```python
from build123d import *

# Parameters (mm, degrees)
SKETCH1_R           = 2.5
BOSS_EXTRUDE5_DEPTH = 2.5
SKETCH7_R           = 20
BOSS_EXTRUDE6_DEPTH = 1.5
CUT_EXTRUDE5_DEPTH  = 3
SKETCH9_R           = 30
SKETCH9_R_2         = 20
BOSS_EXTRUDE8_DEPTH = 2
SKETCH10_R          = 1.5
CUT_EXTRUDE6_DEPTH  = 2
CUT_EXTRUDE7_DEPTH  = 2
FILLET1_R           = 1
FILLET2_R           = 1


# Some blends are built 0.0001 mm under size
with BuildPart() as part:
    # Sketch1 → Boss-Extrude5 (new, symmetric)
    with BuildSketch(Plane.XY):
        Circle(SKETCH1_R)
    extrude(amount=BOSS_EXTRUDE5_DEPTH, both=True)

    # Sketch7 → Boss-Extrude6 (add, symmetric)
    with BuildSketch(Plane.XY):
        Circle(SKETCH7_R)
    extrude(amount=BOSS_EXTRUDE6_DEPTH, both=True)

    # Sketch8 → Cut-Extrude5 (cut)
    with BuildSketch(Plane.XY.offset(1.5)):
        with BuildLine():
            Line((0, 2.5), (0, 17.5))
            ThreePointArc((0, 17.5), (3.385621722, 10), (0, 2.5))
        make_face()
        with BuildLine():
            Line((1.767766953, 1.767766953), (12.374368671, 12.374368671))
            ThreePointArc((12.374368671, 12.374368671), (9.46506389, 4.677071733), (1.767766953, 1.767766953))
        make_face()
        with BuildLine():
            Line((2.5, 0), (17.5, 0))
            ThreePointArc((17.5, 0), (10, -3.385621722), (2.5, 0))
        make_face()
        with BuildLine():
            Line((1.767766953, -1.767766953), (12.374368671, -12.374368671))
            ThreePointArc((12.374368671, -12.374368671), (4.677071733, -9.46506389), (1.767766953, -1.767766953))
        make_face()
        with BuildLine():
            Line((0, -2.5), (0, -17.5))
            ThreePointArc((0, -17.5), (-3.385621722, -10), (0, -2.5))
        make_face()
        with BuildLine():
            Line((-1.767766953, -1.767766953), (-12.374368671, -12.374368671))
            ThreePointArc((-12.374368671, -12.374368671), (-9.46506389, -4.677071733), (-1.767766953, -1.767766953))
        make_face()
        with BuildLine():
            Line((-2.5, 0), (-17.5, 0))
            ThreePointArc((-17.5, 0), (-10, 3.385621722), (-2.5, 0))
        make_face()
        with BuildLine():
            Line((-1.767766953, 1.767766953), (-12.374368671, 12.374368671))
            ThreePointArc((-12.374368671, 12.374368671), (-4.677071733, 9.46506389), (-1.767766953, 1.767766953))
        make_face()
    extrude(amount=-CUT_EXTRUDE5_DEPTH, mode=Mode.SUBTRACT)

    # Sketch9 → Boss-Extrude8 (add, symmetric)
    with BuildSketch(Plane.XY):
        Circle(SKETCH9_R)
        Circle(SKETCH9_R_2, mode=Mode.SUBTRACT)
    extrude(amount=BOSS_EXTRUDE8_DEPTH, both=True)

    # Sketch10 → Cut-Extrude6 (cut)
    with BuildSketch(Plane.XY.offset(2.5)):
        Circle(SKETCH10_R)
    extrude(amount=-CUT_EXTRUDE6_DEPTH, mode=Mode.SUBTRACT)

    # Sketch11 → Cut-Extrude7 (cut)
    with BuildSketch(Plane.XY.offset(0.5)):
        with BuildLine():
            Line((-1.5, 0), (1.5, 0))
            ThreePointArc((1.5, 0), (0, -1.5), (-1.5, 0))
        make_face()
    extrude(amount=-CUT_EXTRUDE7_DEPTH, mode=Mode.SUBTRACT)

    # Fillet1
    fillet1_edges = [part.edges().sort_by_distance(p)[0] for p in [
        (-2.5, 0, -2.5),
    ]]
    fillet(fillet1_edges, radius=FILLET1_R - 0.0001)  # a hair under: the kernel refuses the full size

    # Fillet2
    # the kernel refuses this fillet: 1 mm, written as the material it takes off along each edge
    with BuildSketch(Plane(origin=(0, 0, 2), x_dir=(1, 0, 0), z_dir=(0, -1, 0))) as fillet2_piece_1:
        with BuildLine():
            CenterArc((30 - FILLET2_R, -FILLET2_R), FILLET2_R, 0, 90)
            Line((30 - FILLET2_R, 0), (30 - FILLET2_R, FILLET2_R * 0.02))
            Line((30 - FILLET2_R, FILLET2_R * 0.02), (30 + FILLET2_R * 0.02, FILLET2_R * 0.02))
            Line((30 + FILLET2_R * 0.02, FILLET2_R * 0.02), (30 + FILLET2_R * 0.02, -FILLET2_R))
            Line((30 + FILLET2_R * 0.02, -FILLET2_R), (30, -FILLET2_R))
        make_face()
    revolve(axis=Axis((0, 0, 2), (0, 0, 1)), mode=Mode.SUBTRACT)
    with BuildSketch(Plane(origin=(0, 0, -2), x_dir=(1, 0, 0), z_dir=(0, -1, 0))) as fillet2_piece_2:
        with BuildLine():
            CenterArc((20.866025404, 1), FILLET2_R, 210, 60)
            Line((20.866025404, 0), (20.866025404, -0.02))
            Line((20.866025404, -0.02), (20, -0.02))
            Line((20, -0.02), (19.98, 0))
            ThreePointArc((19.98, 0), (19.98, 0.25), (19.982679492, 0.49))
            Line((19.982679492, 0.49), (20, 0.5))
        make_face()
    revolve(axis=Axis((0, 0, -2), (0, 0, 1)), mode=Mode.SUBTRACT)
    with BuildSketch(Plane(origin=(0, 0, -2), x_dir=(1, 0, 0), z_dir=(0, -1, 0))) as fillet2_piece_3:
        with BuildLine():
            CenterArc((30 - FILLET2_R, FILLET2_R), FILLET2_R, 270, 90)
            Line((30, FILLET2_R), (30 + FILLET2_R * 0.02, FILLET2_R))
            Line((30 + FILLET2_R * 0.02, FILLET2_R), (30 + FILLET2_R * 0.02, -FILLET2_R * 0.02))
            Line((30 + FILLET2_R * 0.02, -FILLET2_R * 0.02), (30 - FILLET2_R, -FILLET2_R * 0.02))
            Line((30 - FILLET2_R, -FILLET2_R * 0.02), (30 - FILLET2_R, 0))
        make_face()
    revolve(axis=Axis((0, 0, -2), (0, 0, 1)), mode=Mode.SUBTRACT)
    with BuildSketch(Plane(origin=(0, 0, 2), x_dir=(1, 0, 0), z_dir=(0, -1, 0))) as fillet2_piece_4:
        with BuildLine():
            CenterArc((20.866025404, -1), FILLET2_R, 90, 60)
            Line((20.866025404, 0), (20.866025404, 0.02))
            Line((20.866025404, 0.02), (20, 0.02))
            Line((20, 0.02), (19.98, 0))
            ThreePointArc((19.98, 0), (19.98, -0.25), (19.982679492, -0.49))
            Line((19.982679492, -0.49), (20, -0.5))
        make_face()
    revolve(axis=Axis((0, 0, 2), (0, 0, 1)), mode=Mode.SUBTRACT)


solid = part.part
```
Here's how the part is built. I have some questions about the finished solid (model axes, mm). A direction names the side the tool comes from. Coordinates: 2 decimals unless noted, no trailing zeros. Return JSON: item names as keys, results as strings. Group by question number.
Item 1: I need wall thicknesses on line 1 (Z direction, x = -22, y = -6); line 2 (Y direction, x = 4, z = -1.8); line 3 (X direction, y = -4.5, z = 1.1). Which ranges of each line are inside material? Lowest first, please. Write a range as from..to.
Item 2: We'd pull the mould along Y, two halves only. Please class faces 5 (the face through (0, 0, -2.5)), 6 (the face through (0, -1, -1.5)), 7 (the face through (7, -7, 0)): +Y half, -Y half, draft (parallel to the pull), parting line (faces both ways), or undercut.
Item 3: On a 3-axis mill with a long thin cutter (end or side, diameter ignored), from which of +Z, -Z, +X, -X, +Y, -Y can I reach the whole of each face in a straight line? I mean faces 1 (the face through (7, 7, 0)), 2 (the face through (0, 1, 0.5)), 3 (the face through (0, -2, 2.5)), 4 (the face through (4.2, 0.3, -1.5)). Say none if no direction works.
Item 4: Will these pins go through, and if not, where does the flat tip stop? P1, Ø1.5, axis at x = -22, y = 21, coming from the +Z side; P2, Ø3, axis at x = -18, y = 0.5, coming from the +Z side; P3, Ø1, axis at x = 0.5, z = 0, coming from the -Y side.
Item 5: If we section it at A-A on y = 9.5: State how many separate pieces and enclosed holes the cut face has, and give its area (3 significant figures).
Calculated:
{
 "1": {"line 1": "z = -2..2", "line 2": "y = -29.33..-19.87, 19.87..29.33", "line 3": "x = -29.66..-9.28, -4.5..-1.74, 0..1.97, 4.5..29.66"},
 "2": {"face 5": "draft", "face 6": "undercut", "face 7": "undercut"},
 "3": {"face 1": "+Z, -Z", "face 2": "+Z", "face 3": "+Z, +X, -X, +Y, -Y", "face 4": "-Z"},
 "4": {"P1": "stops at z = 1.75", "P2": "stops at z = 1.5", "P3": "stops at y = -30"},
 "5": {"separate pieces": "4", "enclosed holes": "0", "area": "159 mm^2"}
}
